Could you check a few things on this model? Use its own coordinates, in mm. Face numbers are marked on the shaded views. A direction names the side the tool comes from. Give positions to 0.01 mm unless a question says otherwise; leave off trailing zeros. Loops run counter-clockwise (first coordinate to the right, second up) from the corner with the lowest first, then second, coordinate; pieces in that order, holes last. Notation, with made-up numbers: (-18, -4.75) -> (16, -4.75) arc R12 cw to (16, 5.25) -> close; hole circle Ø2 at (53.5, 34.25). An arc over 180 degrees is marked (long way). Put each result on its own line as item: value.
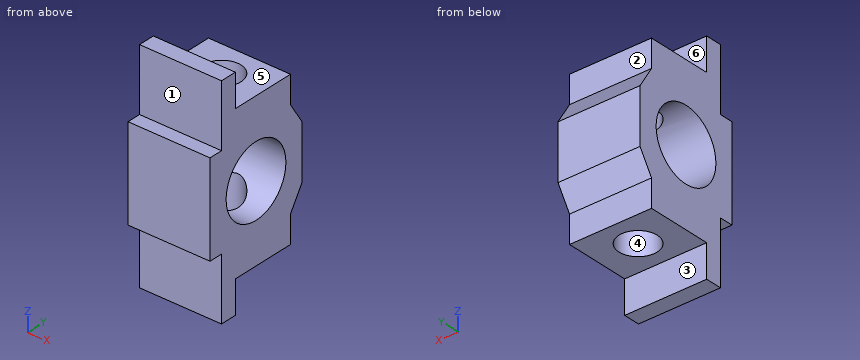
```python
from build123d import *

# Parameters (mm, degrees)
SKETCH1_W           = 30
SKETCH1_H           = 40
BOSS_EXTRUDE1_DEPTH = 40
SKETCH2_W           = 30
SKETCH2_H           = 5
CUT_EXTRUDE1_DEPTH  = 23
SKETCH3_W           = 30
SKETCH3_H           = 5
CUT_EXTRUDE2_DEPTH  = 23
SKETCH5_W           = 12
SKETCH5_H           = 29
CUT_EXTRUDE3_DEPTH  = 65.031242374
CUT_EXTRUDE4_DEPTH  = 65.031242374
SKETCH7_R           = 13
CUT_EXTRUDE5_DEPTH  = 65.031242374
SKETCH8_R           = 7
CUT_EXTRUDE6_DEPTH  = 85.403791384


with BuildPart() as part:
    # Sketch1 → Boss-Extrude1 (new, symmetric)
    with BuildSketch(Plane.XY):
        with Locations((15, 20)):
            Rectangle(SKETCH1_W, SKETCH1_H)
    extrude(amount=BOSS_EXTRUDE1_DEPTH, both=True)

    # Sketch2 → Cut-Extrude1 (cut)
    with BuildSketch(Plane.XY.offset(40)):
        with Locations((15, 2.5)):
            Rectangle(SKETCH2_W, SKETCH2_H)
    extrude(amount=-CUT_EXTRUDE1_DEPTH, mode=Mode.SUBTRACT)

    # Sketch3 → Cut-Extrude2 (cut)
    with BuildSketch(Plane(origin=(0, 0, -40), x_dir=(-1, 0, 0), z_dir=(0, 0, -1))):
        with Locations((-15, 2.5)):
            Rectangle(SKETCH3_W, SKETCH3_H)
    extrude(amount=-CUT_EXTRUDE2_DEPTH, mode=Mode.SUBTRACT)

    # Sketch5 → Cut-Extrude3 (cut, through all)
    with BuildSketch(Plane(origin=(0, 0, 0), x_dir=(0, 0, -1), z_dir=(1, 0, 0))):
        with Locations((-34, 25.5)):
            Rectangle(SKETCH5_W, SKETCH5_H)
        with Locations((34, 25.5)):
            Rectangle(SKETCH5_W, SKETCH5_H)
    extrude(amount=CUT_EXTRUDE3_DEPTH, mode=Mode.SUBTRACT)

    # Sketch6 → Cut-Extrude4 (cut, through all)
    with BuildSketch(Plane(origin=(30, 0, 0), x_dir=(0, 0, -1), z_dir=(1, 0, 0))):
        Polygon((-28, 35), (-18, 35), (-10, 40), (-28, 40), align=None)
        Polygon((10, 40), (18, 35), (28, 35), (28, 40), align=None)
    extrude(amount=-CUT_EXTRUDE4_DEPTH, mode=Mode.SUBTRACT)

    # Sketch7 → Cut-Extrude5 (cut, through all)
    with BuildSketch(Plane(origin=(30, 0, 0), x_dir=(0, 0, -1), z_dir=(1, 0, 0))):
        with Locations((0, 20)):
            Circle(SKETCH7_R)
    extrude(amount=-CUT_EXTRUDE5_DEPTH, mode=Mode.SUBTRACT)

    # Sketch8 → Cut-Extrude6 (cut, through all)
    with BuildSketch(Plane.XY.offset(28)):
        with Locations((15, 23)):
            Circle(SKETCH8_R)
    extrude(amount=-CUT_EXTRUDE6_DEPTH, mode=Mode.SUBTRACT)


solid = part.part
```
1. If we section it at D-D (z = -21.5): List the corners of the cut face in (x, y) for me.
Recorded:
outline: (0, 5) -> (30, 5) -> (30, 35) -> (0, 35) -> close; hole circle Ø14 at (15, 23)
2. I'm going to push flat-ended pins straight in: pin 1 (9.5 mm diameter, centred on x = 15, z = -32.5, fed in from +Y); pin 2 (1.5 mm diameter, centred on x = 22, y = 1.5, fed in from -Z); pin 3 (8 mm diameter, centred on x = 10, y = 23.5, fed in from -Z); pin 4 (2 mm diameter, centred on x = 13, y = 17.5, fed in from -Z) (3 decimals). Where does each tip first touch, or does it pass through?
Recorded:
pin 1: stops at y = 35
pin 2: stops at z = -17
pin 3: stops at z = -28
pin 4: passes through
3. If we section it at B-B (z = 0): List the corners of the cut face in (x, y) for me, then the cut area to 3 significant figures.
Recorded:
outline: (0, 0) -> (30, 0) -> (30, 7) -> (0, 7) -> close; (0, 33) -> (30, 33) -> (30, 40) -> (0, 40) -> close
area: 420 mm^2
4. I need wall thicknesses on line 1 (Y direction, x = 15, z = -21); line 2 (Z direction, x = 23, y = 20); line 3 (X direction, y = 23, z = -21). Which ranges of each line are inside material? Lowest first, please.
Recorded:
line 1: y = 5 to 16, 30 to 35
line 2: z = -28 to -13, 13 to 28
line 3: x = 0 to 8, 22 to 30
5. Thinking about a two-plate mould opening in Y: for the marked faces 4, 5 and 6, which applies, pulls with the +Y half, pulls with the -Y half, needs draft (parallel to the pull), parting line crosses it, or undercut?
Recorded:
face 4: undercut
face 5: needs draft
face 6: pulls with the +Y half
6. If we section it at A-A (x = 23): List the corners of the cut face in (y, z) for me.
Recorded:
outline: (0, -17) -> (5, -17) -> (5, -40) -> (11, -40) -> (11, -28) -> (35, -28) -> (35, -18) -> (40, -10) -> (40, 10) -> (35, 18) -> (35, 28) -> (11, 28) -> (11, 40) -> (5, 40) -> (5, 17) -> (0, 17) -> close; hole circle Ø26 at (20, 0)
7. For the marked faces 1, 2 and 3, which set-ups out of +Z, -Z, +X, -X, +Y, -Y let a thin tool reach every point of the face, with its end or its side?
Recorded:
face 1: +Z, +X, -X, -Y
face 2: +Z, +X, -X, +Y
face 3: -Z, +X, -X, +Y
8. If we section it at C-C (y = 20): List the corners of the cut face in (x, z) for me.
Recorded:
outline: (0, -28) -> (8.68, -28) -> (8.68, -13) -> (0, -13) -> close; (0, 13) -> (8.68, 13) -> (8.68, 28) -> (0, 28) -> close; (21.32, -28) -> (30, -28) -> (30, -13) -> (21.32, -13) -> close; (21.32, 13) -> (30, 13) -> (30, 28) -> (21.32, 28) -> close
